```python
from build123d import *

# Parameters (mm, degrees)
F0_R     = 2.5
F1_DEPTH = 10
F2_W     = 30
F2_H     = 40
F3_DEPTH = 25
F4_R     = 4
F5_DEPTH = 30
F6_W     = 30
F6_H     = 12
F7_DEPTH = 40.001


with BuildPart() as f1:
    # F0 (on Right) → F1 (new body)
    with BuildSketch(Plane.YZ):
        with BuildLine():
            Line((25, 20), (-25, 20))
            ThreePointArc((-25, 20), (-28.535534, 18.535534), (-30, 15))
            Line((-30, 15), (-30, -15))
            ThreePointArc((-30, -15), (-28.535534, -18.535534), (-25, -20))
            Line((-25, -20), (25, -20))
            ThreePointArc((25, -20), (28.535534, -18.535534), (30, -15))
            Line((30, -15), (30, 15))
            ThreePointArc((30, 15), (28.535534, 18.535534), (25, 20))
        make_face()
        with Locations((-22.5, -12.5)):
            Circle(F0_R, mode=Mode.SUBTRACT)
        with Locations((22.5, -12.5)):
            Circle(F0_R, mode=Mode.SUBTRACT)
        with Locations((-22.5, 12.5)):
            Circle(F0_R, mode=Mode.SUBTRACT)
        with Locations((22.5, 12.5)):
            Circle(F0_R, mode=Mode.SUBTRACT)
    extrude(amount=F1_DEPTH)

    # F2 (on face) → F3 (join)
    with BuildSketch(Plane.YZ.offset(10)):
        Rectangle(F2_W, F2_H)
    extrude(amount=F3_DEPTH)

    # F4 (on face) → F5 (cut)
    with BuildSketch(Plane.XZ.offset(15)):
        with BuildLine():
            ThreePointArc((27.977528, 11.235955), (33.099979, 6.624987), (35, 0))
            Line((35, 0), (35, 20))
            Line((35, 20), (10, 20))
            Line((10, 20), (27.977528, 11.235955))
        make_face()
        with BuildLine():
            ThreePointArc((35, 0), (33.099979, -6.624987), (27.977528, -11.235955))
            Line((27.977528, -11.235955), (10, -20))
            Line((10, -20), (35, -20))
            Line((35, -20), (35, 0))
        make_face()
        with Locations((22.5, 0)):
            Circle(F4_R)
    extrude(amount=-F5_DEPTH, mode=Mode.SUBTRACT)

    # F6 (on face) → F7 (cut, through all)
    with BuildSketch(Plane.XY.offset(20)):
        with Locations((25, 0)):
            Rectangle(F6_W, F6_H)
    extrude(amount=-F7_DEPTH, mode=Mode.SUBTRACT)


solid = f1.part
```
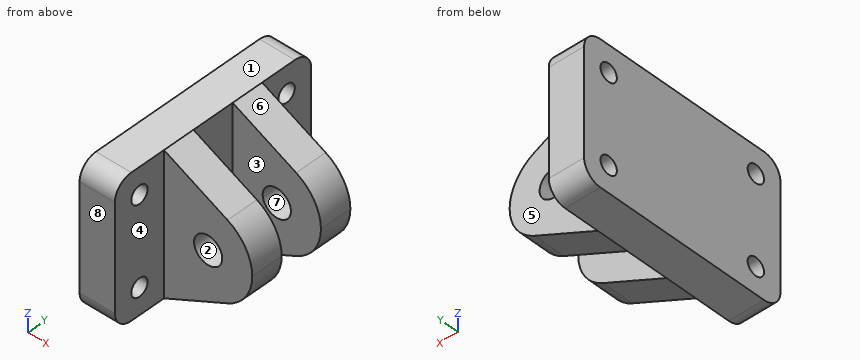
Geometry check sheet. Reference: the model listing, model coordinates, mm. Face numbers are marked on the shaded views. A direction names the side the tool comes from. Coordinates: 2 decimals unless noted, no trailing zeros. Order: outer loops, then holes, each group sorted by start corner. A loop starts at its lowest first (then second) coordinate and runs counter-clockwise, first axis right, second up. Notation, with made-up numbers: (21, -7) - (66, -7) arc R22 cw to (66, 24) - close; hole circle Ø3 at (26.25, 67.25). An arc over 180 degrees is marked (long way). Answer as a JSON object with one key per item and string values. Group by question number.
Item 1: Draft check along Z on the marked faces 6, 7 and 8. Enter one of: +Z half, -Z half, draft (parallel to the pull), parting line (faces both ways), or undercut.
Item 2: Depth check by flat-ended pin: pin 1 Ø6.5 at (y, z) = (-22.5, -12.5) entering from +X; pin 2 Ø9.5 at (y, z) = (-2.5, 5) entering from +X; pin 3 Ø5 at (x, y) = (19.5, -15) entering from -Z. Enter the tip coordinate at first touch or a pass-through.
Item 3: Sectioned sample at C-C, the plane z = -12.5. Record the cut outline in (x, y), and give its area (3 significant figures).
Item 4: Sectioned sample at B-B, the plane x = 3.5. Record the cut outline in (y, z).
Item 5: Scan lines: probe 1 along Y at (x, z) = (19, -15.5); probe 2 along Z at (x, y) = (4.75, 22.5); probe 3 along Z at (x, y) = (3, 22). Record each from-to range of solid material in increasing order.
Item 6: Sectioned sample at D-D, the plane x = 12. Record the cut outline in (y, z) (3 decimals), and give its area (3 significant figures).
Item 7: Tool access check on the marked faces 1, 2, 3, 4 and 5. Record the directions out of +Z, -Z, +X, -X, +Y, -Y that give a thin tool (end or side, any length) a straight path to the whole face; none if there is none.
Item 8: Sectioned sample at A-A, the plane y = 22.5. Record the cut outline in (x, z), and give its area (3 significant figures).
Resolved:
{
 "1": {"face 6": "+Z half", "face 7": "undercut", "face 8": "draft"},
 "2": {"pin 1": "x = 10", "pin 2": "x = 34.87", "pin 3": "z = -16.59"},
 "3": {"outline": "(0, -30) - (10, -30) - (10, -25) - (0, -25) - close; (0, -20) - (10, -20) - (10, -15) - (25.38, -15) - (25.38, -6) - (10, -6) - (10, 6) - (25.38, 6) - (25.38, 15) - (10, 15) - (10, 20) - (0, 20) - close; (0, 25) - (10, 25) - (10, 30) - (0, 30) - close", "area": "777 mm^2"},
 "4": {"outline": "(-30, -15) arc R5 ccw to (-25, -20) - (25, -20) arc R5 ccw to (30, -15) - (30, 15) arc R5 ccw to (25, 20) - (-25, 20) arc R5 ccw to (-30, 15) - close; hole circle Ø5 at (-22.5, -12.5); hole circle Ø5 at (-22.5, 12.5); hole circle Ø5 at (22.5, -12.5); hole circle Ø5 at (22.5, 12.5)"},
 "5": {"probe 1": "-15 to -6, 6 to 15", "probe 2": "-20 to -15, -10 to 10, 15 to 20", "probe 3": "-20 to -14.95, -10.05 to 10.05, 14.95 to 20"},
 "6": {"outline": "(-15, -19.025) - (-6, -19.025) - (-6, 19.025) - (-15, 19.025) - close; (6, -19.025) - (15, -19.025) - (15, 19.025) - (6, 19.025) - close", "area": "685 mm^2"},
 "7": {"face 1": "+Z, +X, -X, +Y, -Y", "face 2": "+Y, -Y", "face 3": "+Z, -Z, +X", "face 4": "+Z, -Z, +X, -Y", "face 5": "+Z, -Z, +X, +Y"},
 "8": {"outline": "(0, -20) - (10, -20) - (10, -15) - (0, -15) - close; (0, -10) - (10, -10) - (10, 10) - (0, 10) - close; (0, 15) - (10, 15) - (10, 20) - (0, 20) - close", "area": "300 mm^2"}
}
